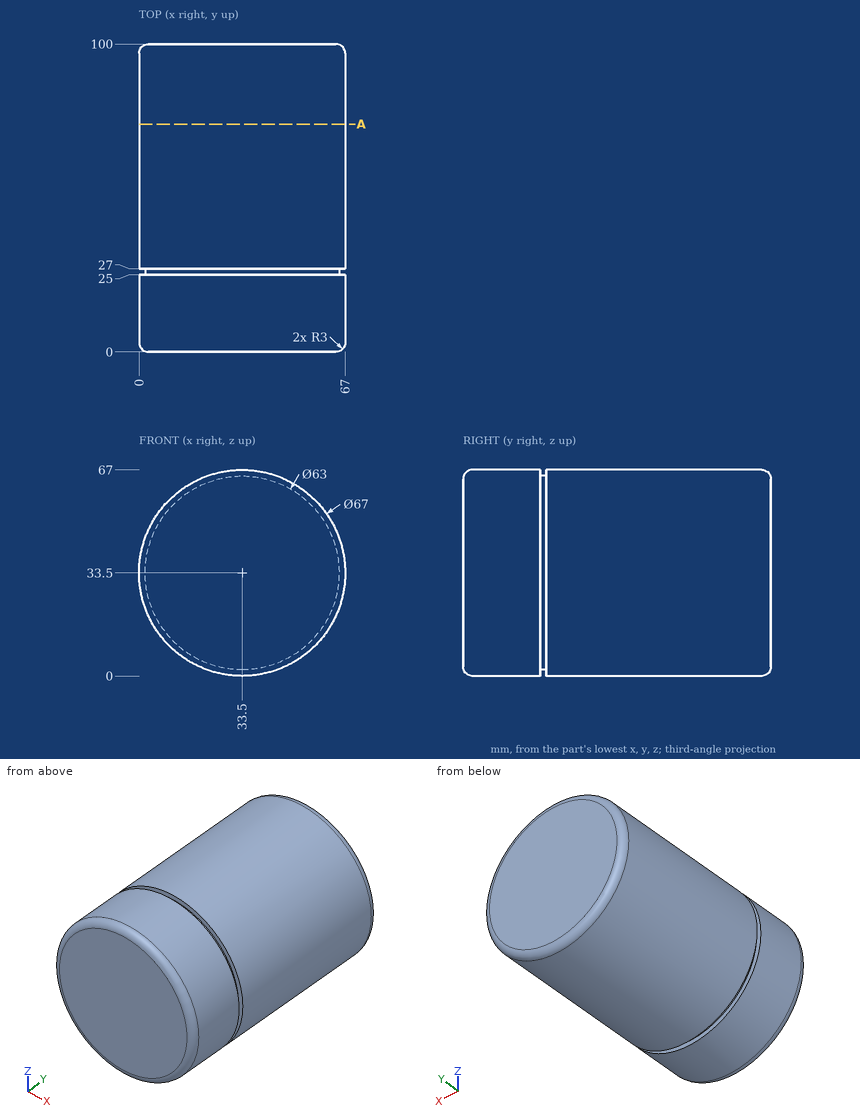
The figure shows three views and two pictorial views of one solid part (mm, origin at its lowest corner). Answer the questions. Round coordinates to 2 decimals unless told otherwise and drop trailing zeros. Write each loop counter-clockwise with the first axis right and the second up, starting at its lowest first coordinate (ties: lowest second). Pieces come first, ordered by that corner, then holes. Notation, with made-up numbers: (85.25, 84.25) - (104.25, 84.25) arc R24 cw to (104.25, 113.25) - close; hole circle Ø9 at (-39, 74.5). An arc over 180 degrees is marked (long way). One line per question, with ' | ' between items. Start each with the question number.
1. Find the intervals of material crossed by probe 1 along Y at (x, z) = (10.5, 57.5); probe 2 along X at (y, z) = (37.5, 34.5); probe 3 along Z at (x, y) = (21.5, 86), in increasing order. Write a range as [from, to].
2. Each of these flat-tipped pins is pushed along its axis until it touches: pin 1 (8 mm diameter, centred on y = 29, z = 11, fed in from -X); pin 2 (8 mm diameter, centred on y = 42, z = 36.5, fed in from -X); pin 3 (2 mm diameter, centred on x = 54.5, y = 76.5, fed in from -Z). Where does it stop, or does it pass through?
3. Section A-A (y = 74) is taken. Determine the outline of the cut face in (x, z), and give its area (3 significant figures).
Filled in:
1) probe 1: [1.78, 25], [27, 98.22] | probe 2: [0.01, 66.99] | probe 3: [2.22, 64.78]
2) pin 1: x = 5.57 | pin 2: x = 0 | pin 3: z = 6.63
3) outline: circle Ø67 at (33.5, 33.5) | area: 3,530 mm²
